Work out the finished part from the listing and answer in its coordinate system (mm). A direction names the side the tool comes from. Round coordinates to 2 decimals unless told otherwise and drop trailing zeros. Loops run counter-clockwise (first coordinate to the right, second up) from the corner with the lowest first, then second, coordinate; pieces in that order, holes last. Notation, with made-up numbers: (76.25, -23) - (114.25, -23) arc R16 ccw to (114.25, -6) - close; hole circle Ø7 at (78.5, 29.25). An arc over 180 degrees is marked (long way). Return JSON: item names as keys, results as strings.
from build123d import *
from OCP.BRepAlgoAPI import BRepAlgoAPI_Cut
from OCP.TopTools import TopTools_ListOfShape

# Parameters (mm, degrees)
BOSS_EXTRUDE1_DEPTH     = 2
SKETCH2_R               = 2.5
BOSS_EXTRUDE2_DEPTH     = 0.666666667
CUT_EXTRUDE1_START      = -4
SKETCH3_R               = 1.25
CUT_EXTRUDE1_DEPTH      = 4
CUT_EXTRUDE3_DEPTH      = 15.256577429
CUT_EXTRUDE3_DEPTH_BACK = 3
BOSS_EXTRUDE3_DEPTH     = 2
CUT_EXTRUDE8_START      = -0.666667
SKETCH7_R               = 2.5
CUT_EXTRUDE8_DEPTH      = 1.333333333
CUT_EXTRUDE9_START      = 2.000000333
SKETCH8_R               = 2.5
CUT_EXTRUDE9_DEPTH      = 1.333333333
SKETCH9_R               = 1.25
CUT_EXTRUDE10_DEPTH     = 5


with BuildPart() as part:
    # Sketch1 → Boss-Extrude1 (new, symmetric)
    with BuildSketch(Plane.XY):
        with BuildLine():
            Line((-8, 0), (-5, 0))
            ThreePointArc((-5, 0), (0, 5), (5, 0))
            Line((5, 0), (8, 0))
            ThreePointArc((8, 0), (1.5281381, 7.85269342), (-7.416198487, 3))
            ThreePointArc((-7.416198487, 3), (-7.85269342, 1.5281381), (-8, 0))
        make_face()
        with BuildLine():
            Line((-13, 0), (-8, 0))
            ThreePointArc((-8, 0), (-7.85269342, 1.5281381), (-7.416198487, 3))
            Line((-7.416198487, 3), (-13, 3))
            Line((-13, 3), (-13, 0))
        make_face()
    extrude(amount=BOSS_EXTRUDE1_DEPTH, both=True)

    # Sketch2 → Boss-Extrude2 (add, symmetric)
    with BuildSketch(Plane.XY):
        with Locations((8, 0)):
            Circle(SKETCH2_R)
    extrude(amount=BOSS_EXTRUDE2_DEPTH, both=True)

    # Sketch3 → Cut-Extrude1 (cut)
    with BuildSketch(Plane.XY.offset(2).offset(CUT_EXTRUDE1_START)):
        with Locations(Location((8, 0, 0), (0, 0, 94.480798786))):
            Circle(SKETCH3_R)
    extrude(amount=CUT_EXTRUDE1_DEPTH, mode=Mode.SUBTRACT)

    # Sketch4 → Cut-Extrude3 (cut, two sides: drawn at the far end of the back side and taken through both)
    with BuildSketch(Plane(origin=(0, 3, 0), x_dir=(1, 0, 0), z_dir=(0, 1, 0)).offset(-CUT_EXTRUDE3_DEPTH_BACK)):
        with BuildLine():
            ThreePointArc((-11, -1.25), (-9.75, 0), (-11, 1.25))
            Line((-11, 1.25), (-13, 1.25))
            Line((-13, 1.25), (-13, -1.25))
            Line((-13, -1.25), (-11, -1.25))
        make_face()
    extrude(amount=CUT_EXTRUDE3_DEPTH + CUT_EXTRUDE3_DEPTH_BACK, mode=Mode.SUBTRACT)

    # Sketch6 → Boss-Extrude3 (add, symmetric)
    with BuildSketch(Plane.XY):
        with BuildLine():
            Line((7.5, 8.5), (-7.5, 8.5))
            Line((-7.5, 8.5), (-7.5, 2.783882181))
            ThreePointArc((-7.5, 2.783882181), (0, 8), (7.5, 2.783882181))
            Line((7.5, 2.783882181), (7.5, 8.5))
        make_face()
    extrude(amount=BOSS_EXTRUDE3_DEPTH, both=True)


with BuildPart() as cut_extrude8_tool:
    # Sketch7 → Cut-Extrude8 (new body)
    with BuildSketch(Plane.XY.offset(CUT_EXTRUDE8_START)):
        with Locations((8, 0)):
            Circle(SKETCH7_R)
    extrude(amount=-CUT_EXTRUDE8_DEPTH)


with BuildPart() as part_1:
    add(part.part)

    # Cut-Extrude8: cut by cut_extrude8_tool, with a tolerance
    cut_extrude8_stock = TopTools_ListOfShape()
    cut_extrude8_stock.Append(part_1.part.wrapped)
    cut_extrude8_tools = TopTools_ListOfShape()
    cut_extrude8_tools.Append(cut_extrude8_tool.part.wrapped)
    cut_extrude8_cut = BRepAlgoAPI_Cut()
    cut_extrude8_cut.SetArguments(cut_extrude8_stock)
    cut_extrude8_cut.SetTools(cut_extrude8_tools)
    cut_extrude8_cut.SetFuzzyValue(0.00001)
    cut_extrude8_cut.Build()
    add(Compound.cast(cut_extrude8_cut.Shape()).solids(), mode=Mode.REPLACE)


with BuildPart() as cut_extrude9_tool:
    # Sketch8 → Cut-Extrude9 (new body)
    with BuildSketch(Plane.XY.offset(CUT_EXTRUDE9_START)):
        with Locations((8, 0)):
            Circle(SKETCH8_R)
    extrude(amount=-CUT_EXTRUDE9_DEPTH)


with BuildPart() as part_2:
    add(part_1.part)

    # Cut-Extrude9: cut by cut_extrude9_tool, with a tolerance
    cut_extrude9_stock = TopTools_ListOfShape()
    cut_extrude9_stock.Append(part_2.part.wrapped)
    cut_extrude9_tools = TopTools_ListOfShape()
    cut_extrude9_tools.Append(cut_extrude9_tool.part.wrapped)
    cut_extrude9_cut = BRepAlgoAPI_Cut()
    cut_extrude9_cut.SetArguments(cut_extrude9_stock)
    cut_extrude9_cut.SetTools(cut_extrude9_tools)
    cut_extrude9_cut.SetFuzzyValue(0.00001)
    cut_extrude9_cut.Build()
    add(Compound.cast(cut_extrude9_cut.Shape()).solids(), mode=Mode.REPLACE)

    # Sketch9 → Cut-Extrude10 (cut)
    with BuildSketch(Plane(origin=(0, 8.5, 0), x_dir=(1, 0, 0), z_dir=(0, 1, 0))):
        with Locations(Location((-5, 0, 0), (0, 0, 180))):
            Circle(SKETCH9_R)
        with Locations(Location((5, 0, 0), (0, 0, 180))):
            Circle(SKETCH9_R)
    extrude(amount=-CUT_EXTRUDE10_DEPTH, mode=Mode.SUBTRACT)


solid = part_2.part
1) Section A-A (z = 1.6) is taken. Give the vertices of the cut face in (x, y), and give its area (3 significant figures).
Verdict:
{"outline": "(-13, 0) - (-5, 0) arc R5 cw to (5, 0) - (5.5, 0) arc R2.5 cw to (7.61, 2.47) arc R8 ccw to (7.5, 2.78) - (7.5, 8.5) - (-7.5, 8.5) - (-7.5, 3) - (-13, 3) - close", "area": "101 mm2"}
2) Flat-ended cylindrical pins translate along their axes: pin 1 (0.7 mm diameter, centred on x = 6.5, y = 1, fed in from +Z); pin 2 (2 mm diameter, centred on y = 3.5, z = -1.5, fed in from +X); pin 3 (1.5 mm diameter, centred on y = 4, z = 0.5, fed in from -X). Find the tip coordinate at first contact, or state that the pin passes through.
Verdict:
{"pin 1": "stops at z = 0.67", "pin 2": "stops at x = 7.6", "pin 3": "stops at x = -7.5"}
3) A tool of negligible diameter and unlimited length cuts with its end or side. For faces 4 (the cylindrical face through (6.115, 1.643, -1.324)), 5 (the flat face through (-7.5, 6, 0)), 6 (the flat face through (-8, 0, 0)), from which of +Z, -Z, +X, -X, +Y, -Y can it reach the whole face along a straight path? Write none if from no direction.
Verdict:
{"face 4": "-Z, +X, -Y", "face 5": "+Z, -Z, -X, +Y", "face 6": "+Z, -Z, -X, -Y"}
4) Section D-D (z = 0) is taken. Give the vertices of the cut face in (x, y).
Verdict:
{"outline": "(-9.75, 0) - (-5, 0) arc R5 cw to (5, 0) - (5.5, 0) arc R2.5 ccw (long way) to (7.61, 2.47) arc R8 ccw to (7.5, 2.78) - (7.5, 8.5) - (6.25, 8.5) - (6.25, 3.5) - (3.75, 3.5) - (3.75, 8.5) - (-3.75, 8.5) - (-3.75, 3.5) - (-6.25, 3.5) - (-6.25, 8.5) - (-7.5, 8.5) - (-7.5, 3) - (-9.75, 3) - close; hole circle Ø2.5 at (8, 0)"}
5) Section C-C (x = 4.75) is taken. Give the vertices of the cut face in (y, z), and give its area (3 significant figures).
Verdict:
{"outline": "(1.56, -2) - (8.5, -2) - (8.5, -1.22) - (3.5, -1.22) - (3.5, 1.22) - (8.5, 1.22) - (8.5, 2) - (1.56, 2) - close", "area": "15.5 mm2"}
6) Section B-B (y = 8) is taken. Give the vertices of the cut face in (x, z).
Verdict:
{"outline": "(-7.5, -2) - (7.5, -2) - (7.5, 2) - (-7.5, 2) - close; hole circle Ø2.5 at (-5, 0); hole circle Ø2.5 at (5, 0)"}
7) Find the intervals of material crossed by L1, parallel to X at y = 6, z = 0.85; L2, parallel to Z at x = -5, y = 4.6; L3, parallel to X at y = 7.5, z = -1.05, in increasing order.
Verdict:
{"L1": "x = -7.5 to -5.92, -4.08 to 4.08, 5.92 to 7.5", "L2": "z = -2 to -1.25, 1.25 to 2", "L3": "x = -7.5 to -5.68, -4.32 to 4.32, 5.68 to 7.5"}
8) Determine the mould class of faces 1 (the cylindrical face through (-3.75, 6.04, 0.05)), 2 (the flat face through (7.5, 6, 0)), 3 (the flat face through (-3, 5, 2)) for opening direction Z: pulls with the +Z half, pulls with the -Z half, needs draft (parallel to the pull), parting line crosses it, or undercut.
Verdict:
{"face 1": "undercut", "face 2": "needs draft", "face 3": "pulls with the +Z half"}
